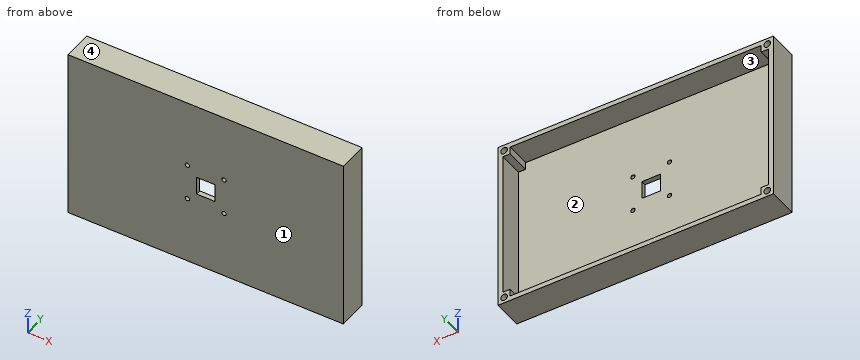
Autodesk Inventor part; units mm, degrees
ref_plane "YZ Plane" through (0, 0, 0) normal (1, 0, 0) x (0, 1, 0)
ref_plane "XZ Plane" through (0, 0, 0) normal (0, 1, 0) x (-1, 0, 0)
ref_plane "XY Plane" through (0, 0, 0) normal (0, 0, 1) x (1, 0, 0)
sketch "Sketch1" plane through (0, 0, 0) normal (0, 1, 0) x (-1, 0, 0)
  line L0 (112.75, -70.75) -> (-112.75, -70.75)
  line L1 (-112.75, -70.75) -> (-112.75, 70.75)
  line L2 (-112.75, 70.75) -> (112.75, 70.75)
  line L3 (112.75, 70.75) -> (112.75, -70.75)
  line L4 (0, -70.75) -> (0, 70.75) construction
  line L5 (112.75, 0) -> (-112.75, 0) construction
  line L6 (112.75, -70.75) -> (102.75, -70.75)
  line L7 (102.75, -66.75) -> (102.75, -60.75)
  line L8 (102.75, -60.75) -> (108.75, -60.75)
  line L9 (112.75, -60.75) -> (112.75, -70.75)
  line L10 (112.75, 70.75) -> (102.75, 70.75)
  line L11 (102.75, 66.75) -> (102.75, 60.75)
  line L12 (102.75, 60.75) -> (108.75, 60.75)
  line L13 (112.75, 60.75) -> (112.75, 70.75)
  line L14 (-112.75, -70.75) -> (-102.75, -70.75)
  line L15 (-102.75, -66.75) -> (-102.75, -60.75)
  line L16 (-102.75, -60.75) -> (-108.75, -60.75)
  line L17 (-112.75, -60.75) -> (-112.75, -70.75)
  line L18 (-102.75, 60.75) -> (-108.75, 60.75)
  line L19 (-112.75, 60.75) -> (-112.75, 70.75)
  line L20 (-112.75, 70.75) -> (-102.75, 70.75)
  line L21 (-102.75, 66.75) -> (-102.75, 60.75)
  line L22 (102.75, -66.75) -> (-102.75, -66.75)
  line L23 (-108.75, -60.75) -> (-108.75, 60.75)
  line L24 (-102.75, 66.75) -> (102.75, 66.75)
  line L25 (108.75, 60.75) -> (108.75, -60.75)
  point P0 (0, 0)
  point P1 (0, 0)
  dimension "d0" = 225.5
  dimension "d1" = 141.5
  dimension "d2" = 10
  dimension "d3" = 10
  dimension "d5" = 4
  dimension "d6" = 4
extrude "Extrusion1" add sketch "Sketch1" along normal blind 24
sketch "Sketch2" plane through (0, 24, 0) normal (0, 1, 0) x (1, 0, 0)
  line L0 (-108.75, 60.75) -> (-102.75, 60.75) construction
  line L1 (-102.75, 60.75) -> (-112.75, 60.75) construction
  line L2 (-112.75, 60.75) -> (-112.75, 70.75) construction
  line L3 (-112.75, 70.75) -> (-102.75, 70.75) construction
  line L4 (-102.75, 70.75) -> (-102.75, 60.75) construction
  line L5 (-112.75, 70.75) -> (-112.75, -70.75) construction
  line L6 (-112.75, 0) -> (112.75, 0) construction
  line L7 (112.75, 70.75) -> (112.75, -70.75) construction
  line L8 (-112.75, -70.75) -> (112.75, -70.75) construction
  line L9 (0, -70.75) -> (0, 70.75) construction
  line L10 (-112.75, 70.75) -> (112.75, 70.75) construction
  circle A0 centre (-107.75, 65.75) radius 2.75
  circle A1 centre (-107.75, -65.75) radius 2.75
  circle A2 centre (107.75, 65.75) radius 2.75
  circle A3 centre (107.75, -65.75) radius 2.75
  point P0 (0, 0)
  dimension "d9" = 5.5
extrude "Extrusion2" cut sketch "Sketch2" against normal blind 7
sketch "Sketch4" plane through (0, 0, 0) normal (0, -1, 0) x (1, 0, 0)
  line L0 (-108.75, -60.75) -> (-108.75, 60.75)
  line L1 (-108.75, 60.75) -> (-102.75, 60.75)
  line L2 (-102.75, 60.75) -> (-102.75, 66.75)
  line L3 (-102.75, 66.75) -> (102.75, 66.75)
  line L4 (102.75, -66.75) -> (-102.75, -66.75)
  line L5 (-102.75, -66.75) -> (-102.75, -60.75)
  line L6 (-102.75, -60.75) -> (-108.75, -60.75)
  line L7 (102.75, -60.75) -> (102.75, -66.75)
  line L8 (108.75, -60.75) -> (102.75, -60.75)
  line L9 (108.75, 60.75) -> (108.75, -60.75)
  line L10 (102.75, 60.75) -> (108.75, 60.75)
  line L11 (102.75, 66.75) -> (102.75, 60.75)
  point P0 (0, 0)
extrude "Extrusion4" add sketch "Sketch4" against normal blind 4
sketch "Sketch5" plane through (0, 0, 0) normal (0, -1, 0) x (1, 0, 0)
  line L0 (112.75, -70.75) -> (-112.75, -70.75) construction
  line L1 (0, -70.75) -> (0, 70.75) construction
  line L2 (-112.75, 70.75) -> (112.75, 70.75) construction
  line L3 (112.75, 70.75) -> (112.75, -70.75) construction
  line L4 (112.75, 0) -> (-112.75, 0) construction
  line L5 (-112.75, -70.75) -> (-112.75, 70.75) construction
  line L6 (0, 0) -> (15, 0) construction
  line L7 (15, 0) -> (15, -15) construction
  line L8 (15, -15) -> (0, -15) construction
  line L9 (0, -15) -> (0, 0) construction
  circle A0 centre (15, -15) radius 1.75
  circle A1 centre (-15, -15) radius 1.75
  circle A2 centre (15, 15) radius 1.75
  circle A3 centre (-15, 15) radius 1.75
  line L10 (7.5, -7.5) -> (-7.5, -7.5)
  line L11 (-7.5, -7.5) -> (-7.5, 7.5)
  line L12 (-7.5, 7.5) -> (7.5, 7.5)
  line L13 (7.5, 7.5) -> (7.5, -7.5)
  dimension "d16" = 15
  dimension "d17" = 15
  dimension "d18" = 3.5
  dimension "d21" = 15
  dimension "d22" = 15
  dimension "d23" = 7.5
  dimension "d24" = 7.5
extrude "Extrusion5" cut sketch "Sketch5" against normal up to next
properties part number "touchscreen_case"
CAD build for the part. Positions are in the model's coordinates, mm. Face numbers are marked on the shaded views. Coordinates: 2 decimals unless noted, no trailing zeros. Write each loop counter-clockwise with the first axis right and the second up, starting at its lowest first coordinate (ties: lowest second). Pieces come first, ordered by that corner, then holes.
(1) Flat gauge pins, fed straight in: pin 1 (4 mm diameter, centred on x = -38, z = 31, fed in from +Y); pin 2 (3 mm diameter, centred on x = 108.5, z = -66, fed in from +Y). Where does each tip first touch, or does it go through?
(2) Cut at A-A, the plane y = 11.5. List the corners of the cut face in (x, z), and give its area (3 significant figures).
(3) Drill centre lines: probe 1 along Z at (x, y) = (-15, 1.35); probe 2 along X at (y, z) = (19, -65.75); probe 3 along Z at (x, y) = (92, 17.75). Where is each one in solid material? Low to high.
(4) Two-plate mould, pull along Z, no slides. Class the marked faces 1, 2, 3 and 4: +Z half, -Z half, draft (parallel to the pull), parting line (faces both ways), or undercut.
(5) Cut at B-B, the plane x = 85.5. List the corners of the cut face in (y, z).
(6) Cut at C-C, the plane z = -25.5. List the corners of the cut face in (x, y).
Geometry says:
1. pin 1: stops at y = 4
1. pin 2: stops at y = 17
2. outline: (-112.75, -70.75) - (112.75, -70.75) - (112.75, 70.75) - (-112.75, 70.75) - close; hole (-108.75, -60.75) - (-102.75, -60.75) - (-102.75, -66.75) - (102.75, -66.75) - (102.75, -60.75) - (108.75, -60.75) - (108.75, 60.75) - (102.75, 60.75) - (102.75, 66.75) - (-102.75, 66.75) - (-102.75, 60.75) - (-108.75, 60.75) - close
2. area: 3,020 mm2
3. probe 1: z = -70.75 to -16.75, -13.25 to 13.25, 16.75 to 70.75
3. probe 2: x = -112.75 to -110.5, -105 to -102.75, 102.75 to 105, 110.5 to 112.75
3. probe 3: z = -70.75 to -66.75, 66.75 to 70.75
4. face 1: draft
4. face 2: undercut
4. face 3: undercut
4. face 4: +Z half
5. outline: (0, -70.75) - (24, -70.75) - (24, -66.75) - (4, -66.75) - (4, 66.75) - (24, 66.75) - (24, 70.75) - (0, 70.75) - close
6. outline: (-112.75, 0) - (112.75, 0) - (112.75, 24) - (108.75, 24) - (108.75, 4) - (-108.75, 4) - (-108.75, 24) - (-112.75, 24) - close
